Autodesk Inventor part; units mm, degrees
ref_plane "YZ Plane" through (0, 0, 0) normal (1, 0, 0) x (0, 1, 0)
ref_plane "XZ Plane" through (0, 0, 0) normal (0, 1, 0) x (-1, 0, 0)
ref_plane "XY Plane" through (0, 0, 0) normal (0, 0, 1) x (1, 0, 0)
sketch "Sketch1" plane through (0, 0, 0) normal (0, 0, 1) x (1, 0, 0)
  arc A0 (-35.4919, 38.1) -> (35.4919, 38.1) centre (0, 0) ccw
  line L0 (-35.4919, 38.1) -> (-73.025, 38.1)
  line L1 (-73.025, 38.1) -> (-73.025, -63.5)
  line L2 (-73.025, -63.5) -> (73.025, -63.5)
  line L3 (73.025, -63.5) -> (73.025, 38.1)
  line L4 (73.025, 38.1) -> (35.4919, 38.1)
  dimension "d0" = 104.14
  dimension "d1" = 146.05
  dimension "d2" = 101.6
  dimension "d3" = 63.5
extrude "Extrusion1" add sketch "Sketch1" along normal blind 25.4
sketch "Sketch3" plane through (-73.025, 38.1, 0) normal (0, 1, 0) x (1, 0, 0)
  line L0 (0, 0) -> (37.5331, 0) construction
  line L1 (0, 0) -> (0, -25.4) construction
  line L2 (37.5331, -25.4) -> (0, -25.4) construction
  line L3 (37.5331, 0) -> (37.5331, -25.4) construction
  line L4 (108.5169, 0) -> (146.05, 0) construction
  line L5 (108.5169, 0) -> (108.5169, -25.4) construction
  line L6 (146.05, -25.4) -> (108.5169, -25.4) construction
  line L7 (146.05, 0) -> (146.05, -25.4) construction
  circle A0 centre (12.7, -12.7) radius 3.4925
  circle A1 centre (133.35, -12.7) radius 3.4925
  point P0 (73.025, 0)
  point P1 (0, -12.7)
  dimension "d6" = 6.985
  dimension "d7" = 6.985
  dimension "d8" = 12.7
  dimension "d9" = 12.7
extrude "Extrusion2" cut sketch "Sketch3" against normal blind 25.4
sketch "Sketch4" plane through (0, 0, 0) normal (0, 0, -1) x (-1, 0, 0)
  arc A0 (-35.4919, 38.1) -> (35.4919, 38.1) centre (0, 0) ccw construction
  line L0 (-35.4919, 38.1) -> (-73.025, 38.1) construction
  line L1 (-73.025, 38.1) -> (-73.025, -63.5) construction
  line L2 (-73.025, -63.5) -> (73.025, -63.5) construction
  line L3 (73.025, -63.5) -> (73.025, 38.1) construction
  line L4 (73.025, 38.1) -> (35.4919, 38.1) construction
  line L5 (-66.04, 30.48) -> (-54.61, 30.48)
  line L6 (-54.61, 30.48) -> (-54.61, 24.13)
  line L7 (-54.61, 24.13) -> (-66.04, 24.13)
  line L8 (-66.04, 24.13) -> (-66.04, 30.48)
  line L9 (-60.325, 30.48) -> (-60.325, 24.13) construction
  dimension "d12" = 11.43
  dimension "d13" = 12.7
  dimension "d14" = 7.62
  dimension "d15" = 6.35
extrude "Extrusion3" cut sketch "Sketch4" against normal blind 20.32
mirror "Mirror1" about plane through (0, 0, 0) normal (1, 0, 0) of "Extrusion3"
fillet "Fillet1" radius 3.175 6 edges at (-35.4919, 38.1, 12.7) (35.4919, 38.1, 12.7) (-73.025, 38.1, 12.7) (-73.025, -63.5, 12.7) (73.025, -63.5, 12.7) (73.025, 38.1, 12.7)
properties part number "Bottom" material "ABS Plastic"
Design review of the part built by this model. Coordinates are the model's own, in mm. A direction names the side the tool comes from. Give positions to 0.01 mm unless a question says otherwise; leave off trailing zeros. Order: outer loops, then holes, each group sorted by start corner. A loop starts at its lowest first (then second) coordinate and runs counter-clockwise, first axis right, second up. Notation, with made-up numbers: (70.25, 76.25) - (92.25, 76.25) arc R29 cw to (92.25, 106.25) - close; hole circle Ø5 at (-32.5, 22). An arc over 180 degrees is marked (long way). Write item = value, one per line. Start each with the question number.
Q1. Mouldability with a two-part tool opening along Y and no side actions: class faces 1 (the face through (60, 30.48, 8)), 2 (the face through (60, 27, 20.32)), 3 (the face through (-72.07, 37.195, 12.878)), 4 (the face through (73.025, -13, 13)) as released by +Y, released by -Y, zero draft, split by the parting line, or undercut.
Q2. To check wall thickness, follow L1, parallel to X at y = 32.75, z = 12.7 (1 decimal); L2, parallel to X at y = 0, z = 8.75 (3 decimals); L3, parallel to X at y = 21.5, z = 12.7 (1 decimal). State the ranges of each line that lie inside material, in increasing order. Write a range as from..to.
Q3. We need section B-B on y = 22. State the section outline as (x, z) points (1 decimal).
Q4. We need section A-A on y = 0. State the section outline as (x, z) points (3 decimals), plus the area to 3 significant figures.
Q5. We need section C-C on z = 5.75. State the section outline as (x, y) points (3 decimals).
Q6. Clearance check with flat-ended pins moving along their axes: pin 1 Ø6 at (x, z) = (-31, 19) entering from +Y; pin 2 Ø1.9 at (x, y) = (62.5, 29) entering from -Z; pin 3 Ø2 at (x, z) = (62, 11) entering from +Y. State where each tip first meets the part, or that it passes through.
Q7. Tool access review of faces 5 (the face through (-39.915, 36.241, 12.878)), 6 (the face through (66.04, 27, 10)), 7 (the face through (63.656, 34.343, 11.651)), 8 (the face through (-1, -57, 25.4)), 9 (the face through (56.5, 38.1, 12.5)): name each direction out of +Z, -Z, +X, -X, +Y, -Y from which nothing blocks a thin tool from reaching the whole face with its end or side.
Q8. We need section D-D on x = -45.5. State the section outline as (y, z) points.
Working result:
q1.face_1 = undercut
q1.face_2 = undercut
q1.face_3 = released by +Y
q1.face_4 = zero draft
q2.L1 = -73..-63.8, -56.8..-40.5, 40.5..56.8, 63.8..73
q2.L2 = -73.025..-52.07, 52.07..73.025
q2.L3 = -73..-63.8, -56.8..-47.4, 47.4..56.8, 63.8..73
q3.outline = (-73, 0) - (-47.2, 0) - (-47.2, 25.4) - (-73, 25.4) - close; (47.2, 0) - (73, 0) - (73, 25.4) - (47.2, 25.4) - close; hole circle Ø7 at (-60.3, 12.7); hole circle Ø7 at (60.3, 12.7)
q4.outline = (-73.025, 0) - (-52.07, 0) - (-52.07, 25.4) - (-73.025, 25.4) - close; (52.07, 0) - (73.025, 0) - (73.025, 25.4) - (52.07, 25.4) - close
q4.area = 1,060 mm²
q5.outline = (-73.025, -60.325) arc R3.175 ccw to (-69.85, -63.5) - (69.85, -63.5) arc R3.175 ccw to (73.025, -60.325) - (73.025, 34.925) arc R3.175 ccw to (69.85, 38.1) - (42.805, 38.1) arc R3.175 ccw to (40.345, 32.918) arc R52.07 cw (long way) to (-40.345, 32.918) arc R3.175 ccw to (-42.805, 38.1) - (-69.85, 38.1) arc R3.175 ccw to (-73.025, 34.925) - close; hole (-66.04, 24.13) - (-54.61, 24.13) - (-54.61, 30.48) - (-66.04, 30.48) - close; hole (54.61, 24.13) - (66.04, 24.13) - (66.04, 30.48) - (54.61, 30.48) - close
q6.pin_1 = -39.44
q6.pin_2 = 20.32
q6.pin_3 = 12.7
q7.face_5 = +Z, -Z
q7.face_6 = -Z
q7.face_7 = +Y
q7.face_8 = +Z, +X, -X, +Y, -Y
q7.face_9 = +Z, -Z, +X, -X, +Y
q8.outline = (-63.5, 0) - (-25.32, 0) - (-25.32, 25.4) - (-63.5, 25.4) - close; (25.32, 0) - (38.1, 0) - (38.1, 25.4) - (25.32, 25.4) - close
